Source: CAD feature listing. Evaluate the final solid. Frame: model axes, mm. Give positions to 0.01 mm unless a question says otherwise; leave off trailing zeros. Order: outer loops, then holes, each group sorted by start corner. A loop starts at its lowest first (then second) coordinate and runs counter-clockwise, first axis right, second up. Notation, with made-up numbers: M -17.75,-20 L 36.25,-20 A12 ccw 36.25,-12 Z; hole C 12,-1.75 d9. An arc over 180 degrees is marked long. Answer as a JSON object with one key per item and string values. Group by question number.
1. Material intervals for L1, parallel to X at y = 2.5, z = 11.25; L2, parallel to X at y = 3.2, z = 41, sorted ascending. Write a range as [from, to].
2. Section query A-A (x = 0). Output: boundary loops of the cut face in (y, z), plus the area to 3 significant figures.
3. Section query C-C (x = -49). Output: boundary loops of the cut face in (y, z), plus the area to 3 significant figures.
4. Pin query (flat end, axial travel): P1, Ø7.5, axis at x = 49.45, z = -16.07, coming from the -Y side; P2, Ø4, axis at x = 17.68, z = -17.68, coming from the +Y side; P3, Ø2, axis at x = -54, y = 0.5, coming from the +Z side; P4, Ø2, axis at x = 26, y = 4.5, coming from the +Z side. Return the tip coordinate at first contact, or that it passes through.
5. Section query B-B (z = 0). Output: boundary loops of the cut face in (x, y).
6. Section query D-D (y = 3.5). Count the separate pieces of the cut face and the enclosed holes in it, plus the area to 3 significant figures.
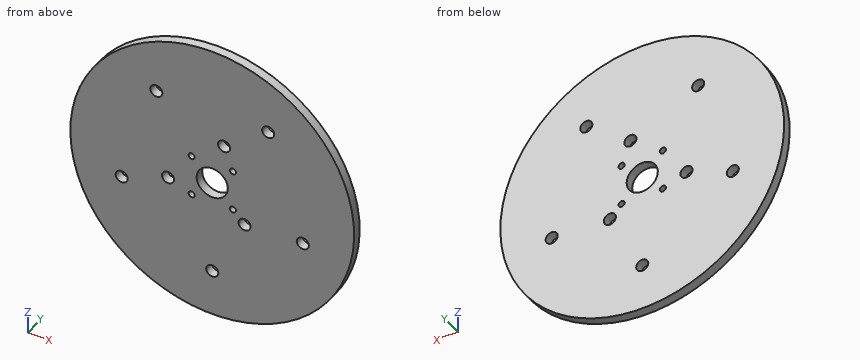
from build123d import *

# Parameters (mm, degrees)
SKETCH1_R            = 77.5
SKETCH1_R_2          = 8.5
BODY_DEPTH           = 5
M6_CLEARANCE_HOLE1_D = 6.6
M3_CLEARANCE_HOLE1_D = 3.4
M6_CLEARANCE_HOLE2_D = 6.6


with BuildPart() as part:
    # Sketch1 → Body (new body)
    with BuildSketch(Plane(origin=(0, 0, 0), x_dir=(1, 0, 0), z_dir=(0, 1, 0))):
        with Locations(Location((0, 0, 0), (0, 0, 270))):
            Circle(SKETCH1_R)
        with Locations(Location((0, 0, 0), (0, 0, 270))):
            Circle(SKETCH1_R_2, mode=Mode.SUBTRACT)
    extrude(amount=BODY_DEPTH)

    # M6 Clearance Hole1 (through all)
    with Locations(Plane(origin=(0, 5, 0), x_dir=(1, 0, 0), z_dir=(0, 1, 0))):
        with Locations((0, 52), (49.454938847, 16.068883707), (30.564833119, -42.068883707), (-30.564833119, -42.068883707), (-49.454938847, 16.068883707), (0, 0)):
            Hole(M6_CLEARANCE_HOLE1_D / 2)

    # M3 Clearance Hole1 (through all)
    with Locations(Plane(origin=(0, 5, 0), x_dir=(1, 0, 0), z_dir=(0, 1, 0))):
        with Locations((0, 0), (-11.25, 11.25), (11.25, -11.25), (11.25, 11.25), (-11.25, -11.25)):
            Hole(M3_CLEARANCE_HOLE1_D / 2)

    # M6 Clearance Hole2 (through all)
    with Locations(Plane(origin=(0, 5, 0), x_dir=(1, 0, 0), z_dir=(0, 1, 0))):
        with Locations((17.67766953, 17.67766953), (6.470476128, -24.148145657), (-24.148145657, 6.470476128), (0, 0)):
            Hole(M6_CLEARANCE_HOLE2_D / 2)


solid = part.part
Answer sheet:
{
 "1": {"L1": "[-76.68, -12.95], [-9.55, 9.55], [12.95, 76.68]", "L2": "[-65.77, -33.69], [-27.44, 27.44], [33.69, 65.77]"},
 "2": {"outline": "M 0,-77.5 L 5,-77.5 L 5,-55.3 L 0,-55.3 Z; M 0,-48.7 L 5,-48.7 L 5,-8.5 L 0,-8.5 Z; M 0,8.5 L 5,8.5 L 5,77.5 L 0,77.5 Z", "area": "657 mm^2"},
 "3": {"outline": "M 0,-60.04 L 5,-60.04 L 5,-19.34 L 0,-19.34 Z; M 0,-12.8 L 5,-12.8 L 5,60.04 L 0,60.04 Z", "area": "568 mm^2"},
 "4": {"P1": "y = 0", "P2": "through", "P3": "z = 56.54", "P4": "z = 73.36"},
 "5": {"outline": "M -77.5,0 L -8.5,0 L -8.5,5 L -77.5,5 Z; M 8.5,0 L 77.5,0 L 77.5,5 L 8.5,5 Z"},
 "6": {"separate pieces": "1", "enclosed holes": "13", "area": "18,300 mm^2"}
}
